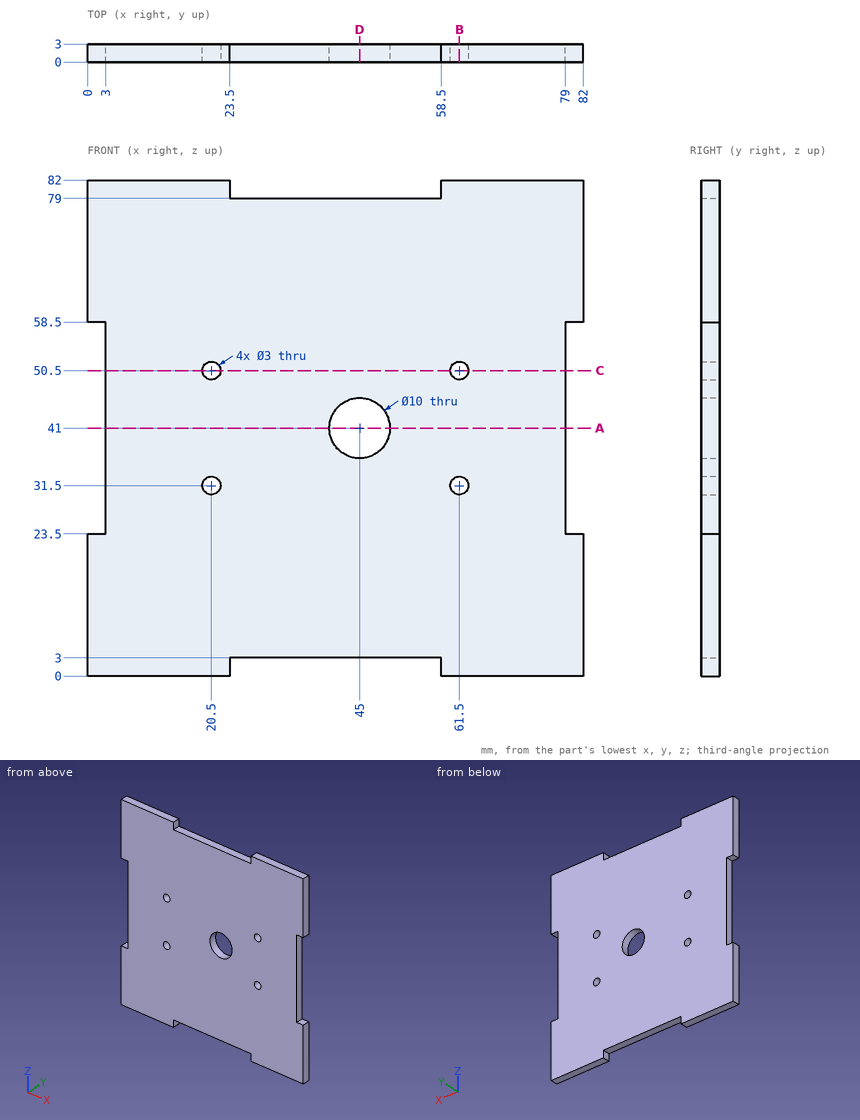
The figure shows three views and two pictorial views of one solid part (mm, origin at its lowest corner). Answer the questions. Give positions to 0.01 mm unless a question says otherwise; leave off trailing zeros. Order: outer loops, then holes, each group sorted by start corner. A loop starts at its lowest first (then second) coordinate and runs counter-clockwise, first axis right, second up. Notation, with made-up numbers: (-12, 27.5) -> (41, 27.5) arc R34 cw to (41, 60.5) -> close; hole circle Ø7 at (70, 46). An arc over 180 degrees is marked (long way). Write each question's results on one line, items separated by ' | '.
Q1. The part is cut by section A-A, the plane z = 41. Give the vertices of the cut face in (x, y), and give its area (3 significant figures).
Checked values:
outline: (3, 0) -> (40, 0) -> (40, 3) -> (3, 3) -> close; (50, 0) -> (79, 0) -> (79, 3) -> (50, 3) -> close | area: 198 mm^2
Q2. Each of these flat-tipped pins is pushed along its axis until it touches: P1, Ø1.5, axis at x = 36, y = 2, coming from the +Z side; P2, Ø1.8, axis at x = 20.5, z = 50.5, coming from the +Y side; P3, Ø1.5, axis at x = 47.5, y = 1, coming from the -Z side. Where does it stop, or does it pass through?
Checked values:
P1: stops at z = 79 | P2: passes through | P3: stops at z = 3
Q3. The part is cut by section C-C, the plane z = 50.5. Give the vertices of the cut face in (x, y), and give its area (3 significant figures).
Checked values:
outline: (3, 0) -> (19, 0) -> (19, 3) -> (3, 3) -> close; (22, 0) -> (60, 0) -> (60, 3) -> (22, 3) -> close; (63, 0) -> (79, 0) -> (79, 3) -> (63, 3) -> close | area: 210 mm^2
Q4. The part is cut by section B-B, the plane x = 61.5. Give the vertices of the cut face in (y, z), and give its area (3 significant figures).
Checked values:
outline: (0, 0) -> (3, 0) -> (3, 30) -> (0, 30) -> close; (0, 33) -> (3, 33) -> (3, 49) -> (0, 49) -> close; (0, 52) -> (3, 52) -> (3, 82) -> (0, 82) -> close | area: 228 mm^2
Q5. Straight lines are drawn through the part: probe 1 along X at (y, z) = (1.85, 50.5); probe 2 along Z at (x, y) = (20.5, 1.35); probe 3 along Z at (x, y) = (30, 1.75). For each, find the intervals that lie inside material, in ascending order. Write a range as from..to.
Checked values:
probe 1: x = 3..19, 22..60, 63..79 | probe 2: z = 0..30, 33..49, 52..82 | probe 3: z = 3..79
Q6. The part is cut by section D-D, the plane x = 45. Give the vertices of the cut face in (y, z), and give its area (3 significant figures).
Checked values:
outline: (0, 3) -> (3, 3) -> (3, 36) -> (0, 36) -> close; (0, 46) -> (3, 46) -> (3, 79) -> (0, 79) -> close | area: 198 mm^2
